Source: CAD feature listing. Evaluate the final solid. Frame: model axes, mm. Face numbers are marked on the shaded views. Round coordinates to 2 decimals unless told otherwise and drop trailing zeros. Order: outer loops, then holes, each group sorted by start corner. A loop starts at its lowest first (then second) coordinate and runs counter-clockwise, first axis right, second up. Notation, with made-up numbers: M -26,70.25 L -18,70.25 A22 cw -18,109.25 Z; hole C 71,-8.75 d1. An arc over 180 degrees is marked long. Use one line per item in the form item = value. Start each with the question number.
Q1. Section B-B (y = -31.5). Return the cut outline in (x, z).
Q2. Pull-direction query (X, two-part tool) for the marked faces 1, 2 and 3; classes: pulls with the +X half, pulls with the -X half, needs draft (parallel to the pull), parting line crosses it, or undercut.
Q3. Material intervals for probe 1 along Z at (x, y) = (0, -0.95); probe 2 along Y at (x, z) = (4, 19); probe 3 along Z at (x, y) = (0, -37.15), sorted ascending.
Q4. Section C-C (y = -24). Return the cut outline in (x, z).
Q5. Contact query for flat-ended pins moving along their axis: pin 1 (5 mm diameter, centred on x = -18.5, y = -9, fed in from -Z); pin 2 (1.5 mm diameter, centred on x = 24, y = -20, fed in from +Z); pin 3 (2 mm diameter, centred on y = -21.5, z = -11.5, fed in from +X); pin 4 (8 mm diameter, centred on x = -7.5, z = 7, fed in from -Y). Output: stop coordinate, or through.
Q6. Section A-A (x = 0). Return the cut outline in (y, z).
from build123d import *

# Parameters (mm, degrees)
F0_R      = 30
F0_R_2    = 27
F1_DEPTH  = 3
F4_R      = 30
F3_R      = 23
F7_R      = 20
F6_R      = 27
F9_R      = 22.403667
F9_R_2    = 12.693191
F10_DEPTH = 2


with BuildPart() as f1:
    # F0 (on Front) → F1 (new body)
    with BuildSketch(Plane.XZ):
        Circle(F0_R)
        Circle(F0_R_2, mode=Mode.SUBTRACT)
    extrude(amount=F1_DEPTH)

    # F4 (on face) → F5 section 0
    with BuildSketch(Plane.XZ.offset(3)):
        Circle(F4_R)
    # F3 (on offset) → F5 section 1
    with BuildSketch(Plane.XZ.offset(38)):
        Circle(F3_R)
    loft()

    # F7 (on face) → F8 section 0
    with BuildSketch(Plane.XZ.offset(38)):
        Circle(F7_R)
    # F6 (on face) → F8 section 1
    with BuildSketch(Plane(origin=(0, -3, 0), x_dir=(-1, 0, 0), z_dir=(0, 1, 0))):
        Circle(F6_R)
    loft(mode=Mode.SUBTRACT)

    # F9 (on face) → F10 (join)
    with BuildSketch(Plane.XZ.offset(38)):
        Circle(F9_R)
        Circle(F9_R_2, mode=Mode.SUBTRACT)
    extrude(amount=-F10_DEPTH)


solid = f1.part
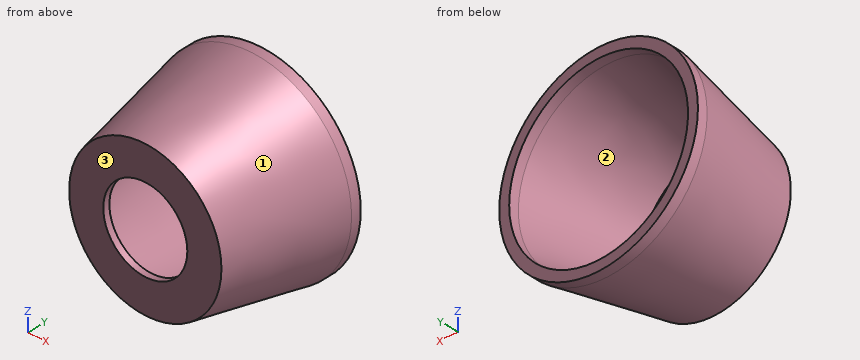
Results list:
q1.outline = C 0,0 d48.6; hole C 0,0 d42.6
q2.face_1 = parting line crosses it
q2.face_2 = undercut
q2.face_3 = needs draft
q3.probe_1 = -30 to -27, 27 to 30
q3.probe_2 = -38 to -36
q3.probe_3 = -23.17 to -12.69, 12.69 to 23.17
q4.outline = C 0,0 d51.6; hole C 0,0 d45.6
q5.pin_1 = -24.05
q5.pin_2 = 12.96
q5.pin_3 = 24.16
q5.pin_4 = -38
q6.outline = M -38,-23 L -3,-30 L 0,-30 L 0,-27 L -3,-27 L -36,-20.4 L -36,-12.69 L -38,-12.69 Z; M -38,12.69 L -36,12.69 L -36,20.4 L -3,27 L 0,27 L 0,30 L -3,30 L -38,23 Z
